For this review, take the finished solid that the model builds, in its own axes (mm). Face numbers are marked on the shaded views. Give positions to 0.01 mm unless a question says otherwise; leave off trailing zeros. Order: outer loops, then holes, each group sorted by start corner. A loop starts at its lowest first (then second) coordinate and runs counter-clockwise, first axis right, second up. Notation, with made-up numbers: (-1.5, 51.25) -> (25.5, 51.25) arc R18 ccw to (25.5, 82.25) -> close; hole circle Ø11 at (-19, 43.25). An arc over 180 degrees is marked (long way). Use CSV: the item, a comma, the result in double quotes. Start each with the question number.
Autodesk Inventor part; units mm, degrees
ref_plane "YZ Plane" through (0, 0, 0) normal (1, 0, 0) x (0, 1, 0)
ref_plane "XZ Plane" through (0, 0, 0) normal (0, 1, 0) x (-1, 0, 0)
ref_plane "XY Plane" through (0, 0, 0) normal (0, 0, 1) x (1, 0, 0)
sketch "Esboço1" plane through (0, 0, 0) normal (1, 0, 0) x (0, 1, 0)
  line L0 (0.4443, 5.6274) -> (-0.9413, 9.5119)
  line L1 (0.4443, 5.6274) -> (-3.3612, 4.0485)
  line L2 (-3.3612, 4.0485) -> (-5.5175, 9.2458)
  line L3 (-5.5175, 9.2458) -> (-5.7078, 6.9431)
  line L4 (-7.3945, -13.4652) -> (7.0591, -13.4652)
  line L5 (7.0591, -13.4652) -> (-5.1461, -7.0903)
  line L6 (-5.1461, -7.0903) -> (0.4923, 3.7048)
  line L7 (0.4923, 3.7048) -> (9.7416, -1.1262)
  arc A0 (-0.9413, 9.5119) -> (9.7416, -1.1262) centre (21.579, 21.4439) ccw
  line L8 (-5.7078, 6.9431) -> (-7.3945, -13.4652)
  point P0 (-0.6447, 8.6807)
extrude "Extrusão1" add sketch "Esboço1" along normal blind 165
properties part number "juncao controle tela"
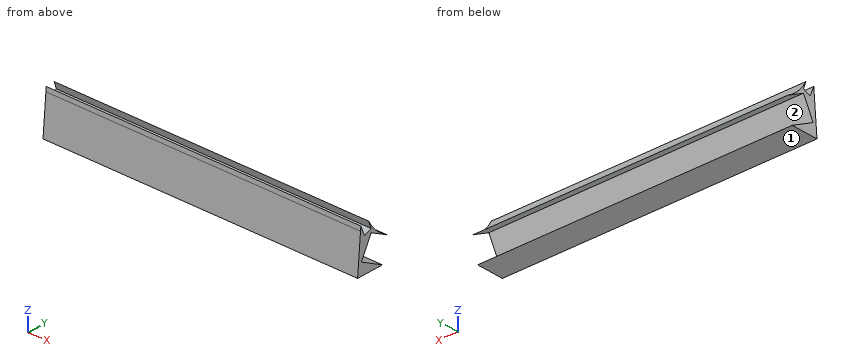
1. Draft analysis for pull direction Z (two halves, no side actions). For the marked faces 1 and 2, state which applies: +Z half, -Z half, draft (parallel to the pull), parting line (faces both ways), or undercut.
2. Consider section A-A (y = 2). State the section outline as (x, z) points.
3. Clearance check with flat-ended pins moving along their axes: P1, Ø8, axis at y = 3, z = -1, coming from the +X side; P2, Ø4, axis at x = 134.5, z = 7, coming from the +Y side; P3, Ø1, axis at x = 94.5, z = -3, coming from the -Y side; P4, Ø2, axis at x = 139.5, z = -4, coming from the -Y side. State where each tip first meets the part, or that it passes through.
4. To check wall thickness, follow L1, parallel to Z at x = 25.5, y = -3; L2, parallel to Z at x = 98, y = -1.25; L3, parallel to Y at x = 147.5, z = -10. State the ranges of each line that lie inside material, in increasing order. Write a range as [from, to].
5. Consider section B-B (x = 25.5). State the section outline as (y, z) points.
Answer list:
1,face 1,"-Z half"
1,face 2,"undercut"
2,outline,"(0, -13.47) -> (165, -13.47) -> (165, -10.82) -> (0, -10.82) -> close; (0, 2.92) -> (165, 2.92) -> (165, 5.13) -> (0, 5.13) -> close"
3,P1,"x = 165"
3,P2,"y = 2.11"
3,P3,"y = -6.57"
3,P4,"y = -6.69"
4,L1,"[-13.47, -8.21], [-2.98, 4.2]"
4,L2,"[-13.47, -9.13], [0.37, 4.92]"
4,L3,"[-7.11, 0.42]"
5,outline,"(-7.39, -13.47) -> (7.06, -13.47) -> (-5.15, -7.09) -> (0.49, 3.7) -> (9.74, -1.13) arc R25.49 cw to (-0.94, 9.51) -> (0.44, 5.63) -> (-3.36, 4.05) -> (-5.52, 9.25) -> (-5.71, 6.94) -> close"
